Could you check a few things on this drawing? It's one solid part, dimensions in mm from its lowest x, y, z. Give positions to 0.01 mm unless a question says otherwise; leave off trailing zeros. Loops run counter-clockwise (first coordinate to the right, second up) from the corner with the lowest first, then second, coordinate; pieces in that order, holes last. Notation, with made-up numbers: M -8.5,57.5 L 28.5,57.5 A19 cw 28.5,71.5 Z; hole C 87.5,31 d7. An arc over 180 degrees is marked long. Write each question's results on one line, items separated by ' | '. Start each with the question number.
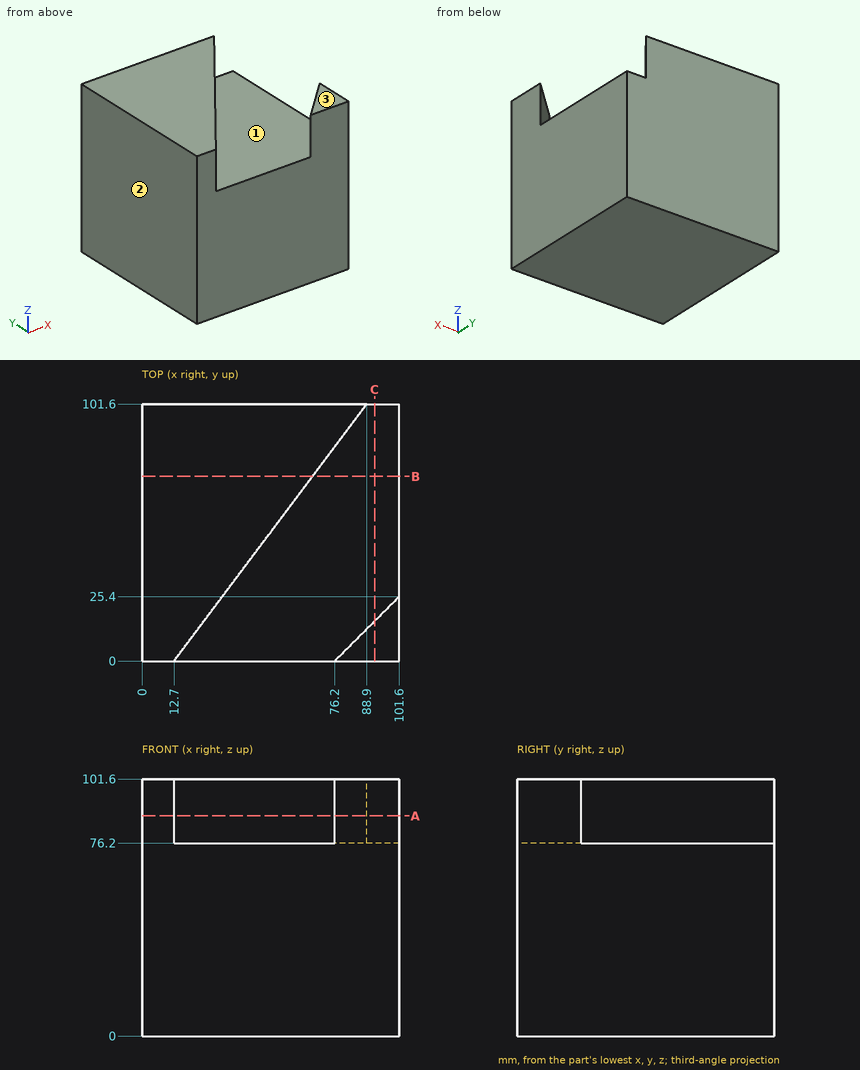
1) If we section it at B-B on y = 73: Write out the boundary of the cut face in (x, z), plus the area to 3 significant figures.
2) If we section it at C-C on x = 92: Write out the boundary of the cut face in (y, z), plus the area to 3 significant figures.
3) Please list where these lines run through material, in increasing order: line 1 (Z direction, x = 91.5, y = 93); line 2 (X direction, y = 12, z = 95); line 3 (X direction, y = 13, z = 89). Write a range as from..to.
4) I'm going to push flat-ended pins straight in: P1, Ø12, axis at x = 91, y = 36.5, coming from the +Z side; P2, Ø12, axis at y = 48, z = 85.5, coming from the +X side. Where does each tip first touch, or does it pass through?
5) Thinking about a two-plate mould opening in X: for the marked faces 1, 2 and 3, which applies, pulls with the +X half, pulls with the -X half, needs draft (parallel to the pull), parting line crosses it, or undercut?
6) If we section it at A-A on z = 87: Write out the boundary of the cut face in (x, y), plus the area to 3 significant figures.
Calculated:
1) outline: M 0,0 L 101.6,0 L 101.6,76.2 L 67.45,76.2 L 67.45,101.6 L 0,101.6 Z | area: 9,460 mm2
2) outline: M 0,0 L 101.6,0 L 101.6,76.2 L 15.8,76.2 L 15.8,101.6 L 0,101.6 Z | area: 8,140 mm2
3) line 1: z = 0..76.2 | line 2: x = 0..21.7, 88.2..101.6 | line 3: x = 0..22.45, 89.2..101.6
4) P1: stops at z = 76.2 | P2: stops at x = 53.2
5) face 1: undercut | face 2: pulls with the -X half | face 3: needs draft
6) outline: M 0,0 L 12.7,0 L 88.9,101.6 L 0,101.6 Z; M 76.2,0 L 101.6,0 L 101.6,25.4 Z | area: 5,480 mm2
